from build123d import *

# Parameters (mm, degrees)
SKETCH1_R                    = 54.1
SKETCH1_R_2                  = 3.175
BOSS_EXTRUDE1_DEPTH          = 35
BOSS_EXTRU_3_START           = -35
BOSS_EXTRU_3_DEPTH           = 20
R_P_TITION_CIRCULAIRE3_COUNT = 3
BOSS_EXTRU_4_START           = -55
ESQUISSE3_R                  = 3.175
BOSS_EXTRU_4_DEPTH           = 55
R_P_TITION_CIRCULAIRE4_COUNT = 3
ECHELLE1_SCALE               = 2


with BuildPart() as part:
    # Sketch1 → Boss-Extrude1 (new body)
    with BuildSketch(Plane.XY):
        Circle(SKETCH1_R)
        with Locations((0, 30.75)):
            Circle(SKETCH1_R_2, mode=Mode.SUBTRACT)
        with Locations((26.630281166, -15.375)):
            Circle(SKETCH1_R_2, mode=Mode.SUBTRACT)
        with Locations((-26.630281166, -15.375)):
            Circle(SKETCH1_R_2, mode=Mode.SUBTRACT)
        Circle(SKETCH1_R_2, mode=Mode.SUBTRACT)
        with BuildLine():
            Line((-3.175, 4.719838451), (-3.175, 21.514108743))
            ThreePointArc((-3.175, 21.514108743), (-4.149238079, 23.494525508), (-6.312640449, 23.931424332))
            ThreePointArc((-6.312640449, 23.931424332), (-21.434128744, 12.375), (-23.881541645, -6.498805172))
            ThreePointArc((-23.881541645, -6.498805172), (-22.421474979, -8.153917171), (-20.219264711, -8.007423714))
            Line((-20.219264711, -8.007423714), (-5.675, 0.389711432))
            ThreePointArc((-5.675, 0.389711432), (-3.844872981, 2.219838451), (-3.175, 4.719838451))
        make_face(mode=Mode.SUBTRACT)
        with BuildLine():
            Line((3.175, 4.719838451), (3.175, 21.514108743))
            ThreePointArc((3.175, 21.514108743), (4.149238079, 23.494525508), (6.312640449, 23.931424332))
            ThreePointArc((6.312640449, 23.931424332), (21.434128744, 12.375), (23.881541645, -6.498805172))
            ThreePointArc((23.881541645, -6.498805172), (22.421474979, -8.153917171), (20.219264711, -8.007423714))
            Line((20.219264711, -8.007423714), (5.675, 0.389711432))
            ThreePointArc((5.675, 0.389711432), (3.844872981, 2.219838451), (3.175, 4.719838451))
        make_face(mode=Mode.SUBTRACT)
        with BuildLine():
            Line((2.5, -5.109549882), (17.044264711, -13.506685028))
            ThreePointArc((17.044264711, -13.506685028), (18.2722369, -15.340608337), (17.568901196, -17.43261916))
            ThreePointArc((17.568901196, -17.43261916), (0, -24.75), (-17.568901196, -17.43261916))
            ThreePointArc((-17.568901196, -17.43261916), (-18.2722369, -15.340608337), (-17.044264711, -13.506685028))
            Line((-17.044264711, -13.506685028), (-2.5, -5.109549882))
            ThreePointArc((-2.5, -5.109549882), (0, -4.439676901), (2.5, -5.109549882))
        make_face(mode=Mode.SUBTRACT)
    extrude(amount=BOSS_EXTRUDE1_DEPTH)

    # Esquisse1 → Boss.-Extru.3 (add)
    with BuildSketch(Plane.XY.offset(35).offset(BOSS_EXTRU_3_START)):
        with BuildLine():
            Line((-21.394470874, 15.186776811), (-23.849369957, 10.934766872))
            ThreePointArc((-23.849369957, 10.934766872), (-25.80163538, 9.32891658), (-28.328409714, 9.4031251))
            ThreePointArc((-28.328409714, 9.4031251), (-29.704475683, 9.828675415), (-31.133898102, 10.005881992))
            ThreePointArc((-31.133898102, 10.005881992), (-32.768655428, 10.889813252), (-33.053443696, 12.726294025))
            Line((-33.053443696, 12.726294025), (-30.300729733, 17.494134468))
            Line((-30.300729733, 17.494134468), (-27.548015769, 22.261974911))
            ThreePointArc((-27.548015769, 22.261974911), (-25.815182633, 22.933581423), (-24.232297044, 21.959805679))
            ThreePointArc((-24.232297044, 21.959805679), (-23.364120437, 20.81049284), (-22.307550068, 19.831559912))
            ThreePointArc((-22.307550068, 19.831559912), (-20.979896438, 17.680413408), (-21.394470874, 15.186776811))
        make_face()
    boss_extru_3 = extrude(amount=-BOSS_EXTRU_3_DEPTH)

    # Répétition circulaire3: Boss.-Extru.3 ×3 about axis
    r_p_tition_circulaire3_axis = Axis((0, 0, 0), (0, 0, 1))
    for i in range(1, R_P_TITION_CIRCULAIRE3_COUNT):
        add(boss_extru_3.rotate(r_p_tition_circulaire3_axis, i * 360 / R_P_TITION_CIRCULAIRE3_COUNT))

    # Esquisse3 → Boss.-Extru.4 (add)
    with BuildSketch(Plane.XY.offset(35).offset(BOSS_EXTRU_4_START)):
        with Locations((0, 30.75)):
            Circle(ESQUISSE3_R)
    boss_extru_4 = extrude(amount=BOSS_EXTRU_4_DEPTH)

    # Répétition circulaire4: Boss.-Extru.4 ×3 about axis
    r_p_tition_circulaire4_axis = Axis((0, 0, 0), (0, 0, 1))
    for i in range(1, R_P_TITION_CIRCULAIRE4_COUNT):
        add(boss_extru_4.rotate(r_p_tition_circulaire4_axis, i * 360 / R_P_TITION_CIRCULAIRE4_COUNT))


with BuildPart() as part_1:
    # Echelle1: scaled about (0, 0, 16.669882878)
    add(part.part.scale(ECHELLE1_SCALE).moved(Location((0, 0, -16.669882878))))


solid = part_1.part
Part model, mm, in its own coordinate system. A direction names the side the tool comes from. Give positions to 0.01 mm unless a question says otherwise; leave off trailing zeros. Loops run counter-clockwise (first coordinate to the right, second up) from the corner with the lowest first, then second, coordinate; pieces in that order, holes last.
(1) 3-axis set-ups, long thin cutter, end or side, ignore diameter. For faces 1 (the flat face through (-26.098, -7.735, 17.84)), 2 (the cylindrical face through (-51.68, 45.87, -36.39)), 3 (the cylindrical face through (41.946, 35.29, -36.39)): which of +Z, -Z, +X, -X, +Y, -Y reach the whole face in a straight line?
Return value:
face 1: +Z, -Z
face 2: -Z, +Y
face 3: -Z
(2) Band-saw the part on B-B (z = -10). Write the cut outline in (x, y), and give its area (3 significant figures).
Return value:
outline: circle Ø216.4 at (0, 0); hole (-47.76, -13) arc R5 ccw to (-40.44, -16.01) - (-11.35, 0.78) arc R10 ccw to (-6.35, 9.44) - (-6.35, 43.03) arc R5 ccw to (-12.63, 47.86) arc R49.5 ccw to start; hole (-35.14, -34.87) arc R49.5 ccw to (35.14, -34.87) arc R5 ccw to (34.09, -27.01) - (5, -10.22) arc R10 ccw to (-5, -10.22) - (-34.09, -27.01) arc R5 ccw to start; hole circle Ø12.7 at (0, 0); hole (6.35, 9.44) arc R10 ccw to (11.35, 0.78) - (40.44, -16.01) arc R5 ccw to (47.76, -13) arc R49.5 ccw to (12.63, 47.86) arc R5 ccw to (6.35, 43.03) - close
area: 30,800 mm2
(3) Drill centre lines: line 1 along Y through (x, z) = (0, -1); line 2 along X through (y, z) = (19.5, 1.5); line 3 along Z through (x, y) = (16, -52.5). Where is each one in solid material? Low to high.
Return value:
line 1: y = -108.2 to -49.5, -8.88 to -6.35, 6.35 to 108.2
line 2: x = -106.43 to -45.5, -6.35 to 6.35, 45.5 to 106.43
line 3: z = -16.67 to 53.33
(4) Pull direction Y, two halves, no side cores. Call faces 4 (the flat face through (-53, -31, -56.67)), 5 (the flat face through (26.098, -7.735, 17.84)), 6 (the cylindrical face through (12.67, -61.24, -36.39)), 7 (the cylindrical face through (65.568, 21.824, -36.39)): pulls with the +Y half, pulls with the -Y half, needs draft (parallel to the pull), parting line crosses it, or undercut.
Return value:
face 4: needs draft
face 5: undercut
face 6: pulls with the +Y half
face 7: parting line crosses it
(5) Band-saw the part on C-C (z = -45). Write the cut outline in (x, y).
Return value:
outline: (-66.11, 25.45) arc R4.18 ccw to (-62.27, 20.01) arc R16.34 cw to (-56.66, 18.81) arc R7.2 ccw to (-47.7, 21.87) - (-42.79, 30.37) arc R7.2 ccw to (-44.62, 39.66) arc R16.34 cw to (-48.46, 43.92) arc R4.18 ccw to (-55.1, 44.52) - close; circle Ø12.7 at (-53.26, -30.75); (-13.8, -63.93) arc R4.18 ccw to (-11.01, -69.98) - (11.01, -69.98) arc R4.18 ccw to (13.8, -63.93) arc R16.34 cw to (12.04, -58.47) arc R7.2 ccw to (4.91, -52.24) - (-4.91, -52.24) arc R7.2 ccw to (-12.04, -58.47) arc R16.34 cw to start; circle Ø12.7 at (0, 61.5); (42.79, 30.37) - (47.7, 21.87) arc R7.2 ccw to (56.66, 18.81) arc R16.34 cw to (62.27, 20.01) arc R4.18 ccw to (66.11, 25.45) - (55.1, 44.52) arc R4.18 ccw to (48.46, 43.92) arc R16.34 cw to (44.62, 39.66) arc R7.2 ccw to start; circle Ø12.7 at (53.26, -30.75)
(6) Band-saw the part on D-D (y = 61.5). Write the cut outline in (x, z).
Return value:
outline: (-89.02, -16.67) - (-6.35, -16.67) - (-6.35, -56.67) - (6.35, -56.67) - (6.35, -16.67) - (89.02, -16.67) - (89.02, 53.33) - (-89.02, 53.33) - close
(7) Band-saw the part on A-A (y = -40). Write the cut outline in (x, z).
Return value:
outline: (-100.53, -16.67) - (-29.16, -16.67) - (-29.16, 53.33) - (-100.53, 53.33) - close; (29.16, -16.67) - (100.53, -16.67) - (100.53, 53.33) - (29.16, 53.33) - close
(8) Pin check, flat tips, straight feed: pin 1 (5 mm diameter, centred on x = -42, y = 48.5, fed in from -Z); pin 2 (8 mm diameter, centred on x = 24.5, z = 12, fed in from -Y); pin 3 (2 mm diameter, centred on y = -39.5, z = -3, fed in from -X). Stop position of each tip, or through.
Return value:
pin 1: stops at z = -16.67
pin 2: stops at y = -106.24
pin 3: stops at x = -101.12
